For this review, take the finished solid that the model builds, in its own axes (mm). Give positions to 0.01 mm unless a question says otherwise; leave off trailing zeros. Loops run counter-clockwise (first coordinate to the right, second up) from the corner with the lowest first, then second, coordinate; pieces in that order, holes last. Notation, with made-up numbers: (18.5, 71.25) - (35.5, 71.25) arc R18 ccw to (35.5, 88.25) - close; hole circle Ø2 at (55.5, 22). An arc over 180 degrees is marked (long way). Put each result on its own line as item: value.
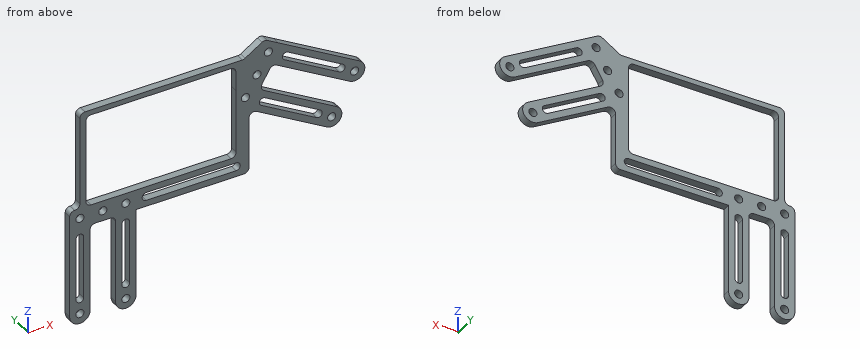
from build123d import *

# Parameters (mm, degrees)
SKETCH1_R           = 1.6
BOSS_EXTRUDE1_DEPTH = 3
FILLET1_R           = 2
FILLET2_R           = 2
CUT_EXTRUDE1_DEPTH  = 3
BOSS_EXTRUDE2_DEPTH = 3
SKETCH5_W           = 5.72828372
SKETCH5_H           = 7.781232697
CUT_EXTRUDE2_DEPTH  = 3
SKETCH6_R           = 1.6
CUT_EXTRUDE3_DEPTH  = 3
FILLET3_R           = 2
CUT_EXTRUDE4_DEPTH  = 3


with BuildPart() as part:
    # Sketch1 → Boss-Extrude1 (new body)
    # profile 1 of 3: a face of its own
    with BuildSketch(Plane(origin=(0, 0, 0), x_dir=(1, 0, 0), z_dir=(0, 1, 0))):
        Polygon((66.235042478, 4), (-4, 4), (-4, -4), (61.235042478, -4), (61.235042478, -28.773130918), (72.398403011, -48.108638544), (79.326606241, -44.108638544), (66.235042478, -21.433384956), align=None)
        with Locations(Location((18, 0, 0), (0, 0, 270))):
            Circle(SKETCH1_R, mode=Mode.SUBTRACT)
        with Locations(Location((9, 0, 0), (0, 0, 270))):
            Circle(SKETCH1_R, mode=Mode.SUBTRACT)
        with Locations(Location((0, 0, 0), (0, 0, 270))):
            Circle(SKETCH1_R, mode=Mode.SUBTRACT)
        with Locations(Location((64.862504626, -27.056079661, 0), (0, 0, 270))):
            Circle(SKETCH1_R, mode=Mode.SUBTRACT)
        with Locations(Location((69.362504626, -34.850308295, 0), (0, 0, 270))):
            Circle(SKETCH1_R, mode=Mode.SUBTRACT)
        with Locations(Location((73.862504626, -42.644536929, 0), (0, 0, 270))):
            Circle(SKETCH1_R, mode=Mode.SUBTRACT)
    # profile 2 of 3: a face of its own
    with BuildSketch(Plane(origin=(0, 0, 0), x_dir=(1, 0, 0), z_dir=(0, 1, 0))):
        Polygon((2.360744243, -4), (0, -4), (0, -42.879937828), (64.221215797, -42.879937828), (61.09340732, -40.879937828), (2.360744243, -40.879937828), align=None)
    # profile 3 of 3: a face of its own
    with BuildSketch(Plane(origin=(0, 0, 0), x_dir=(1, 0, 0), z_dir=(0, 1, 0))):
        Polygon((61.235042478, -28.773130918), (72.398403011, -48.108638544), (61.09340732, -40.879937828), align=None)
    extrude(amount=BOSS_EXTRUDE1_DEPTH)

    # Fillet1
    fillet1_edges = [part.edges().sort_by_distance(p)[0] for p in [
        (61.235042478, 1.5, 28.773130918),
        (61.235042478, 1.5, 4),
        (2.360744243, 1.5, 4),
        (2.360744243, 1.5, 40.879937828),
        (61.09340732, 1.5, 40.879937828),
    ]]
    fillet(fillet1_edges, radius=FILLET1_R)

    # Fillet2
    fillet2_edges = [part.edges().sort_by_distance(p)[0] for p in [
        (0, 1.5, 4),
        (-4, 1.5, 4),
        (-4, 1.5, -4),
        (66.235042478, 1.5, -4),
        (66.235042478, 1.5, 21.433384956),
        (79.326606241, 1.5, 44.108638544),
        (72.398403011, 1.5, 48.108638544),
        (64.221215797, 1.5, 42.879937828),
        (0, 1.5, 42.879937828),
    ]]
    fillet(fillet2_edges, radius=FILLET2_R - 0.0001)  # a hair under: the kernel refuses the full size

    # Sketch2 → Cut-Extrude1 (cut)
    with BuildSketch(Plane(origin=(0, 3, 0), x_dir=(1, 0, 0), z_dir=(0, 1, 0))):
        with BuildLine():
            Line((26, 1.6), (61.235042478, 1.6))
            ThreePointArc((61.235042478, 1.6), (62.835042478, 0), (61.235042478, -1.6))
            Line((61.235042478, -1.6), (26, -1.6))
            ThreePointArc((26, -1.6), (24.4, 0), (26, 1.6))
        make_face()
    extrude(amount=-CUT_EXTRUDE1_DEPTH, mode=Mode.SUBTRACT)

    # Sketch4 → Boss-Extrude2 (add)
    with BuildSketch(Plane(origin=(0, 3, 0), x_dir=(1, 0, 0), z_dir=(0, 1, 0))):
        with BuildLine():
            Line((-2.0001, 4), (4, 4))
            Line((4, 4), (4, 39))
            ThreePointArc((4, 39), (0, 43), (-4, 39))
            Line((-4, 39), (-4, 2.0001))
            ThreePointArc((-4, 2.0001), (-3.414242852, 3.414242852), (-2.0001, 4))
        make_face()
        with BuildLine():
            Line((14, 39), (14, 4))
            Line((14, 4), (22, 4))
            Line((22, 4), (22, 39))
            ThreePointArc((22, 39), (18, 43), (14, 39))
        make_face()
        with BuildLine():
            Line((96.637495374, -4.091978046), (66.35375998, -21.576300827))
            ThreePointArc((66.35375998, -21.576300827), (66.421246357, -21.740191472), (66.502978273, -21.897463366))
            Line((66.502978273, -21.897463366), (70.326606241, -28.520181276))
            Line((70.326606241, -28.520181276), (100.637495374, -11.020181276))
            ThreePointArc((100.637495374, -11.020181276), (102.101596989, -5.556079661), (96.637495374, -4.091978046))
        make_face()
        with BuildLine():
            Line((105.637495374, -19.680435314), (75.326606241, -37.180435314))
            Line((75.326606241, -37.180435314), (78.326656241, -42.376674339))
            ThreePointArc((78.326656241, -42.376674339), (78.526447096, -43.894236547), (77.594642036, -45.108588544))
            Line((77.594642036, -45.108588544), (109.637495374, -26.608638544))
            ThreePointArc((109.637495374, -26.608638544), (111.101596989, -21.144536929), (105.637495374, -19.680435314))
        make_face()
    extrude(amount=-BOSS_EXTRUDE2_DEPTH)

    # Sketch5 → Cut-Extrude2 (cut)
    with BuildSketch(Plane(origin=(0, 3, 0), x_dir=(1, 0, 0), z_dir=(0, 1, 0))):
        with Locations((58.370900618, -27.25388929)):
            Rectangle(SKETCH5_W, SKETCH5_H)
    extrude(amount=-CUT_EXTRUDE2_DEPTH, mode=Mode.SUBTRACT)

    # Sketch6 → Cut-Extrude3 (cut)
    with BuildSketch(Plane(origin=(0, 3, 0), x_dir=(1, 0, 0), z_dir=(0, 1, 0))):
        with Locations(Location((0, 39, 0), (0, 0, 270))):
            Circle(SKETCH6_R)
        with Locations(Location((18, 39, 0), (0, 0, 270))):
            Circle(SKETCH6_R)
        with Locations(Location((98.637495374, -7.556079661, 0), (0, 0, 270))):
            Circle(SKETCH6_R)
        with Locations(Location((107.637495374, -23.144536929, 0), (0, 0, 270))):
            Circle(SKETCH6_R)
    extrude(amount=-CUT_EXTRUDE3_DEPTH, mode=Mode.SUBTRACT)

    # Fillet3
    fillet3_edges = [part.edges().sort_by_distance(p)[0] for p in [
        (14, 1.5, -4),
        (4, 1.5, -4),
        (75.326606241, 1.5, 37.180435314),
        (70.326606241, 1.5, 28.520181276),
        (66.35375998, 1.5, 21.576300827),
    ]]
    fillet(fillet3_edges, radius=FILLET3_R)

    # Sketch8 → Cut-Extrude4 (cut)
    with BuildSketch(Plane(origin=(0, 3, 0), x_dir=(1, 0, 0), z_dir=(0, 1, 0))):
        with BuildLine():
            Line((1.5, 33), (1.5, 8))
            ThreePointArc((1.5, 8), (0, 6.5), (-1.5, 8))
            Line((-1.5, 8), (-1.5, 33))
            ThreePointArc((-1.5, 33), (0, 34.5), (1.5, 33))
        make_face()
        with BuildLine():
            Line((19.5, 33), (19.5, 8))
            ThreePointArc((19.5, 8), (18, 6.5), (16.5, 8))
            Line((16.5, 8), (16.5, 33))
            ThreePointArc((16.5, 33), (18, 34.5), (19.5, 33))
        make_face()
        with BuildLine():
            Line((94.191342951, -11.855117767), (72.540707856, -24.355117767))
            ThreePointArc((72.540707856, -24.355117767), (70.491669751, -23.806079661), (71.040707856, -21.757041555))
            Line((71.040707856, -21.757041555), (92.691342951, -9.257041555))
            ThreePointArc((92.691342951, -9.257041555), (94.740381057, -9.806079661), (94.191342951, -11.855117767))
        make_face()
        with BuildLine():
            Line((103.191342951, -27.443575035), (81.540707856, -39.943575035))
            ThreePointArc((81.540707856, -39.943575035), (79.491669751, -39.394536929), (80.040707856, -37.345498823))
            Line((80.040707856, -37.345498823), (101.691342951, -24.845498823))
            ThreePointArc((101.691342951, -24.845498823), (103.740381057, -25.394536929), (103.191342951, -27.443575035))
        make_face()
    extrude(amount=-CUT_EXTRUDE4_DEPTH, mode=Mode.SUBTRACT)


solid = part.part
1) Wall thickness on line 1 (X direction, y = 1.4, z = 0); line 2 (X direction, y = 1.45, z = -26); line 3 (Z direction, x = 30, y = 2.7): over which ranges is each line inside the solid? List them lowest first.
Geometry check:
line 1: x = -4 to -1.6, 1.6 to 7.4, 10.6 to 16.4, 19.6 to 24.4, 62.84 to 66.24
line 2: x = -4 to -1.5, 1.5 to 4, 14 to 16.5, 19.5 to 22
line 3: z = -4 to -1.6, 1.6 to 4, 40.88 to 42.88
2) Insertion check: pin 1 Ø1.5 at (x, y) = (52, 1.5) entering from -Z; pin 2 Ø1.5 at (x, y) = (68.5, 2.5) entering from +Z; pin 3 Ø0.9 at (y, z) = (1.5, 22.5) entering from -X. Each pin has a flat end and moves straight along its axis. Give the tip position at first contact, or say it passes through.
Geometry check:
pin 1: stops at z = -4
pin 2: stops at z = 46.1
pin 3: stops at x = 0
3) Take a section at D-D on y = 1.5. State how many separate pieces and enclosed holes the cut face has, and give its area (3 significant figures).
Geometry check:
separate pieces: 1
enclosed holes: 16
area: 1,840 mm²
4) Take a section at A-A on x = 45.5. State the section outline as (y, z) points, and give its area (3 significant figures).
Geometry check:
outline: (0, -4) - (3, -4) - (3, -1.6) - (0, -1.6) - close; (0, 1.6) - (3, 1.6) - (3, 4) - (0, 4) - close; (0, 40.88) - (3, 40.88) - (3, 42.88) - (0, 42.88) - close
area: 20.4 mm²
5) Take a section at B-B on z = -20.5. State the section outline as (x, y) points, and give its area (3 significant figures).
Geometry check:
outline: (-4, 0) - (-1.5, 0) - (-1.5, 3) - (-4, 3) - close; (1.5, 0) - (4, 0) - (4, 3) - (1.5, 3) - close; (14, 0) - (16.5, 0) - (16.5, 3) - (14, 3) - close; (19.5, 0) - (22, 0) - (22, 3) - (19.5, 3) - close
area: 30.0 mm²
6) Take a section at C-C on z = 0. State the section outline as (x, y) points, and give its area (3 significant figures).
Geometry check:
outline: (-4, 0) - (-1.6, 0) - (-1.6, 3) - (-4, 3) - close; (1.6, 0) - (7.4, 0) - (7.4, 3) - (1.6, 3) - close; (10.6, 0) - (16.4, 0) - (16.4, 3) - (10.6, 3) - close; (19.6, 0) - (24.4, 0) - (24.4, 3) - (19.6, 3) - close; (62.84, 0) - (66.24, 0) - (66.24, 3) - (62.84, 3) - close
area: 66.6 mm²
